Here's how the part is built. I have some questions about the finished solid (model axes, mm). Face numbers are marked on the shaded views. A direction names the side the tool comes from. Give positions to 0.01 mm unless a question says otherwise; leave off trailing zeros. Write each loop counter-clockwise with the first axis right and the second up, starting at its lowest first coordinate (ties: lowest second). Pieces come first, ordered by that corner, then holes. Notation, with made-up numbers: M 77,88 L 112,88 A33 cw 112,121 Z; hole C -39,54.25 d2. An arc over 180 degrees is marked long. Use one line per item in the form item = value. Start each with the question number.
from build123d import *

# Parameters (mm, degrees)
SKETCH_W        = 64
SKETCH_H        = 21
PAD_DEPTH       = 25
SKETCH001_W     = 62
SKETCH001_H     = 19
POCKET_DEPTH    = 24
SKETCH003_R     = 3.25
POCKET001_DEPTH = 5
SKETCH004_R     = 2
PAD001_DEPTH    = 3.5
SKETCH005_W     = 20
SKETCH005_H     = 1
PAD002_DEPTH    = 63
CHAMFER_SIZE    = 3.4
SKETCH006_R     = 1.5
PAD003_DEPTH    = 10
SKETCH007_R     = 0.5
POCKET002_DEPTH = 8
CHAMFER001_SIZE = 1.4


with BuildPart() as part:
    # Sketch → Pad (new body)
    with BuildSketch(Plane.XY):
        with Locations((32, 10.5)):
            Rectangle(SKETCH_W, SKETCH_H)
    extrude(amount=PAD_DEPTH)

    # Sketch001 (on Face6 of Pad) → Pocket (cut)
    with BuildSketch(Plane.XY.offset(25)):
        with Locations((33, 10.5)):
            Rectangle(SKETCH001_W, SKETCH001_H)
    extrude(amount=-POCKET_DEPTH, mode=Mode.SUBTRACT)

    # Sketch003 (on Face10 of Pocket) → Pocket001 (cut)
    with BuildSketch(Plane.YZ.offset(2)):
        with Locations((10.5, 7)):
            Circle(SKETCH003_R)
    extrude(amount=-POCKET001_DEPTH, mode=Mode.SUBTRACT)

    # Sketch004 (on Face9 of Pocket001) → Pad001 (join)
    with BuildSketch(Plane.XY.offset(1)):
        with Locations((15, 10.5)):
            Circle(SKETCH004_R)
        with Locations((50, 10.5)):
            Circle(SKETCH004_R)
    extrude(amount=PAD001_DEPTH)

    # Sketch005 (on Face3 of Pad001) → Pad002 (join)
    with BuildSketch(Plane.YZ.offset(64)):
        with Locations((10.5, 24.5)):
            Rectangle(SKETCH005_W, SKETCH005_H)
    extrude(amount=-PAD002_DEPTH)

    # Chamfer
    chamfer_edges = [part.edges().sort_by_distance(p)[0] for p in [
        (13, 10.5, 1),
        (48, 10.5, 1),
    ]]
    chamfer(chamfer_edges, length=CHAMFER_SIZE)

    # Sketch006 (on Face5 of Chamfer) → Pad003 (join)
    with BuildSketch(Plane.YZ.offset(64)):
        with Locations((1.5, 23.5)):
            Circle(SKETCH006_R)
        with Locations((19.5, 23.5)):
            Circle(SKETCH006_R)
        with Locations((1.5, 1.5)):
            Circle(SKETCH006_R)
        with Locations((19.5, 1.5)):
            Circle(SKETCH006_R)
    extrude(amount=-PAD003_DEPTH)

    # Sketch007 → Pocket002 (cut)
    with BuildSketch(Plane.YZ.offset(64)):
        with Locations((1.5, 23.5)):
            Circle(SKETCH007_R)
        with Locations((19.5, 23.5)):
            Circle(SKETCH007_R)
        with Locations((1.5, 1.5)):
            Circle(SKETCH007_R)
        with Locations((19.5, 1.5)):
            Circle(SKETCH007_R)
    extrude(amount=-POCKET002_DEPTH, mode=Mode.SUBTRACT)

    # Chamfer001
    chamfer001_edges = [part.edges().sort_by_distance(p)[0] for p in [
        (54, 1.957107, 1),
        (54, 1, 1.957107),
        (54, 20, 1.957107),
        (54, 19.042893, 1),
        (54, 1, 23.042893),
        (54, 1.957107, 24),
        (54, 19.042893, 24),
        (54, 20, 23.042893),
    ]]
    chamfer(chamfer001_edges, length=CHAMFER001_SIZE)


solid = part.part
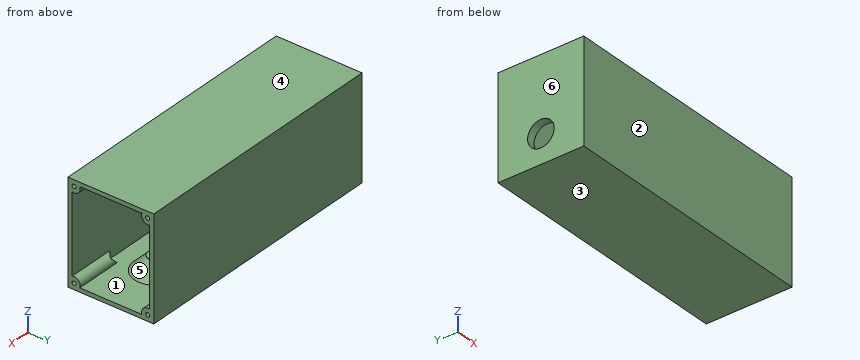
1) On a 3-axis mill with a long thin cutter (end or side, diameter ignored), from which of +Z, -Z, +X, -X, +Y, -Y can I reach the whole of each face in a straight line? I mean the marked faces 5 and 6. Say none if no direction works.
2) Thinking about a two-plate mould opening in Z: for the marked faces 1, 2, 3 and 4, which applies, released by +Z, released by -Z, zero draft, split by the parting line, or undercut?
3) Suppose I cut it at D-D, the plane z = 18.5. List the corners of the cut face in (x, y) for me.
4) Please list where these lines run through material, in increasing order: line 1 (Z direction, x = 59.5, y = 19.5); line 2 (Z direction, x = 33, y = 19.75); line 3 (Z direction, x = 0.6, y = 10.5).
5) Suppose I cut it at B-B, the plane x = 28.5. List the corners of the cut face in (y, z) for me, and give its area (3 significant figures).
6) Suppose I cut it at C-C, the plane z = 7. List the corners of the cut face in (x, y) for me, and give its area (3 significant figures).
7) Suppose I cut it at A-A, the plane y = 10.5. List the corners of the cut face in (x, z) for me, and give its area (3 significant figures).
8) Will this pin go through, and if not, where does the flat tip stop? P1, Ø0.5, axis at y = 19.5, z = 1.5, coming from the +X side.
Checks:
q1.face_5 = none
q1.face_6 = +Z, -Z, -X, +Y, -Y
q2.face_1 = undercut
q2.face_2 = zero draft
q2.face_3 = released by -Z
q2.face_4 = released by +Z
q3.outline = M 0,0 L 64,0 L 64,1 L 2,1 L 2,20 L 64,20 L 64,21 L 0,21 Z
q4.line_1 = 0 to 1, 2 to 3, 22 to 23, 24 to 25
q4.line_2 = 0 to 1, 24 to 25
q4.line_3 = 0 to 3.75, 10.25 to 25
q5.outline = M 0,0 L 21,0 L 21,25 L 0,25 Z; hole M 1,1 L 20,1 L 20,24 L 1,24 Z
q5.area = 88.0 mm^2
q6.outline = M 0,0 L 64,0 L 64,1 L 2,1 L 2,7.25 L 0,7.25 Z; M 0,13.75 L 2,13.75 L 2,20 L 64,20 L 64,21 L 0,21 Z
q6.area = 153 mm^2
q7.outline = M 0,0 L 64,0 L 64,1 L 55.4,1 L 52,4.4 L 52,4.5 L 48,4.5 L 48,4.4 L 44.6,1 L 20.4,1 L 17,4.4 L 17,4.5 L 13,4.5 L 13,4.4 L 9.6,1 L 2,1 L 2,3.75 L 0,3.75 Z; M 0,10.25 L 2,10.25 L 2,24 L 64,24 L 64,25 L 0,25 Z
q7.area = 212 mm^2
q8.P1 = 56
